Work out the finished part from the listing and answer in its coordinate system (mm). Give positions to 0.01 mm unless a question says otherwise; leave off trailing zeros. Loops run counter-clockwise (first coordinate to the right, second up) from the corner with the lowest first, then second, coordinate; pieces in that order, holes last. Notation, with made-up numbers: (62, 0) - (69, 0) arc R12 ccw to (69, 10) - close; hole circle Ø8 at (34, -26.5). An arc over 180 degrees is marked (long way). One line per item, written item: value.
Autodesk Inventor part; units mm, degrees
ref_plane "YZ Plane" through (0, 0, 0) normal (1, 0, 0) x (0, 1, 0)
ref_plane "XZ Plane" through (0, 0, 0) normal (0, 1, 0) x (-1, 0, 0)
ref_plane "XY Plane" through (0, 0, 0) normal (0, 0, 1) x (1, 0, 0)
sketch "Эскиз3" plane through (0, 0, 0) normal (0, 0, 1) x (1, 0, 0)
  circle A0 centre (-21, 40.5) radius 2.7
  line L0 (0, 0) -> (8.3957, 0)
  line L1 (0, 0) -> (0, -7.8184)
  circle A1 centre (21, 40.5) radius 2.7
  circle A2 centre (-21, -40.5) radius 2.7
  circle A3 centre (21, -40.5) radius 2.7
  circle A4 centre (-21, 25) radius 1.75
  circle A5 centre (21, 25) radius 1.75
  circle A6 centre (-21, -25) radius 1.75
  circle A7 centre (21, -25) radius 1.75
  line L2 (-26.5, 40.332) -> (-26.5, 0)
  arc A8 (-21.3, 45.6934) -> (-26.5, 40.332) centre (-21, 40.2) ccw
  line L3 (-21.3, 45.6934) -> (-12.5, 45.6934)
  line L4 (-12.5, 45.6934) -> (-12.5, 48.9877)
  arc A9 (0, 49.934) -> (-12.5, 48.9877) centre (0, -33.098) ccw
  line L5 (-26.5, -40.332) -> (-26.5, 0)
  arc A10 (-26.5, -40.332) -> (-21.3, -45.6934) centre (-21, -40.2) ccw
  line L6 (-21.3, -45.6934) -> (-12.5, -45.6934)
  line L7 (-12.5, -45.6934) -> (-12.5, -48.9877)
  arc A11 (-12.5, -48.9877) -> (0, -49.934) centre (0, 33.098) ccw
  line L8 (26.5, 40.332) -> (26.5, 0)
  arc A12 (26.5, 40.332) -> (21.3, 45.6934) centre (21, 40.2) ccw
  line L9 (21.3, 45.6934) -> (12.5, 45.6934)
  line L10 (12.5, 45.6934) -> (12.5, 48.9877)
  arc A13 (12.5, 48.9877) -> (0, 49.934) centre (0, -33.098) ccw
  line L11 (26.5, -40.332) -> (26.5, 0)
  arc A14 (21.3, -45.6934) -> (26.5, -40.332) centre (21, -40.2) ccw
  line L12 (21.3, -45.6934) -> (12.5, -45.6934)
  arc A15 (0, -49.934) -> (12.5, -48.9877) centre (0, 33.098) ccw
  line L13 (12.5, -45.6934) -> (12.5, -48.9877)
  circle A16 centre (-10, 38.5) radius 1.75
  circle A17 centre (10, 38.5) radius 1.75
  circle A18 centre (-10, -38.5) radius 1.75
  circle A19 centre (10, -38.5) radius 1.75
  dimension "d19" = 5.4
  dimension "d20" = 42
  dimension "d21" = 81
  dimension "d22" = 3.5
  dimension "d23" = 42
  dimension "d24" = 50
  dimension "d25" = 0
  dimension "d26" = 53
  dimension "d27" = 0.168
  dimension "d28" = 0
  dimension "d29" = 0.3
  dimension "d31" = 12.5
  dimension "d32" = 73.298
  dimension "d33" = 83.032
  dimension "d34" = 0
  dimension "d35" = 0.3
  dimension "d38" = 3.5
  dimension "d39" = 20
  dimension "d40" = 77
extrude "Тело" add sketch "Эскиз3" along normal blind 1 contours A8 L3 L4 A9 A13 L10 L9 A12 L8 L11 A14 L12 L13 A15 A11 L7 L6 A10 L5 L2 | A16 | A17 | A18 | A19
properties part number "board_outline"
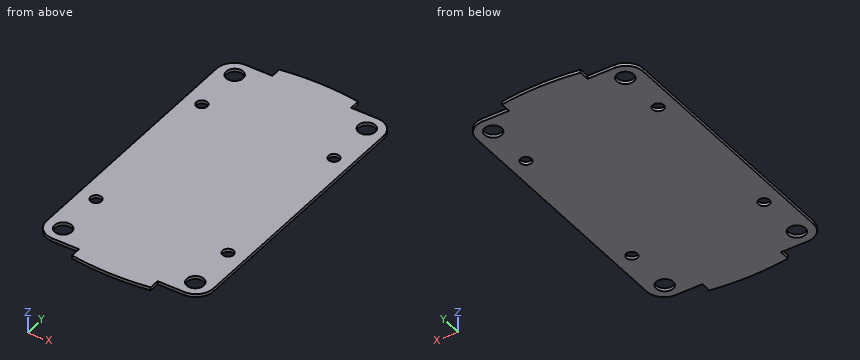
1. Find the intervals of material crossed by line 1 along Y through (x, z) = (21, 0.45); line 2 along Y through (x, z) = (19.5, 0.1) (3 decimals); line 3 along Y through (x, z) = (23, 0.15), in increasing order.
Output:
line 1: y = -45.69 to -43.2, -37.8 to -26.75, -23.25 to 23.25, 26.75 to 37.8, 43.2 to 45.69
line 2: y = -45.693 to -42.745, -38.255 to -25.901, -24.099 to 24.099, 25.901 to 38.255, 42.745 to 45.693
line 3: y = -45.33 to -42.31, -38.69 to 38.69, 42.31 to 45.33
2. Section B-B (z = 0.15) is taken. Count the separate pieces of the cut face and the enclosed holes in it, and give its area (3 significant figures).
Output:
separate pieces: 1
enclosed holes: 8
area: 4,880 mm²
3. Flat-ended cylindrical pins translate along their axes: pin 1 Ø0.5 at (y, z) = (-46.5, 0.5) entering from -X; pin 2 Ø0.5 at (x, z) = (16, 0.5) entering from +Y. Find the tip coordinate at first contact, or state that the pin passes through.
Output:
pin 1: stops at x = -12.5
pin 2: stops at y = 45.69
4. Section A-A (y = 25) is taken. Write down the section's boundary in (x, z), and give its area (3 significant figures).
Output:
outline: (-26.5, 0) - (-22.75, 0) - (-22.75, 1) - (-26.5, 1) - close; (-19.25, 0) - (19.25, 0) - (19.25, 1) - (-19.25, 1) - close; (22.75, 0) - (26.5, 0) - (26.5, 1) - (22.75, 1) - close
area: 46.0 mm²
